Input: part model. Units: mm. Frame: model coordinates. A direction names the side the tool comes from. Coordinates: 2 decimals unless noted, no trailing zeros. Write each loop counter-clockwise with the first axis right and the second up, starting at its lowest first coordinate (ties: lowest second). Pieces come first, ordered by that corner, then holes. Notation, with made-up numbers: (-36.5, -12) - (5.5, -12) arc R23 cw to (5.5, 0) - close; hole circle Ø1 at (25, 50). An arc over 180 degrees is marked (long way). Use a Markdown table: item, result. Add a question column.
Q1. Pin query (flat end, axial travel): P1, Ø7.5, axis at x = 6, y = -5, coming from the -Z side. Return the tip coordinate at first contact, or that it passes through.
Q2. Material intervals for probe 1 along X at (y, z) = (-23.5, 1.35); probe 2 along Y at (x, z) = (6, 1.2); probe 3 along Y at (x, z) = (26, 2.1), sorted ascending. Write a range as from..to.
Q3. Set-up query: faces 5 (the face through (1, -42, 1)), 6 (the face through (23, -12, 1)), 7 (the face through (12.341, -22.308, 2.065)). Return all of +Z, -Z, +X, -X, +Y, -Y with unobstructed straight access to the full face (end or side cutting, diameter ignored); none if empty.
Q4. Section query A-A (z = 0.4). Return the cut outline in (x, y), then the cut area to 3 significant figures.
Q5. Section query B-B (y = -19). Return the cut outline in (x, z).
Q6. Section query C-C (x = 6). Return the cut outline in (y, z).
Q7. Mould query, pull axis Y, two halves, no side actions, for faces 1 (the face through (16, -44, 1)), 2 (the face through (17.8, -21.7, 2.6)), 3 (the face through (1, -2, 1)), 4 (the face through (18.6, -12.57, 1.32)). Classes: released by +Y, released by -Y, zero draft, split by the parting line, or undercut.
Q8. Section query D-D (x = 18.5). Return the cut outline in (y, z), then the cut area to 3 significant figures.
from build123d import *

# Parameters (mm, degrees)
F0_W     = 32
F0_H     = 44
F1_DEPTH = 2.6
F2_R     = 2.35
F3_DEPTH = 2.6
F5_DEPTH = 44.001
F6_R     = 5
F8_DEPTH = 2.601


with BuildPart() as f1:
    # F0 (on Top) → F1 (new body)
    with BuildSketch(Plane.XY):
        with Locations((16, -22)):
            Rectangle(F0_W, F0_H)
    extrude(amount=F1_DEPTH)

    # F2 (on face) → F3 (cut, through all)
    with BuildSketch(Plane.XY.offset(2.6)):
        with Locations((6, -5)):
            Circle(F2_R)
        with Locations((6, -39)):
            Circle(F2_R)
        with Locations((26, -39)):
            Circle(F2_R)
        with Locations((26, -5)):
            Circle(F2_R)
    extrude(amount=-F3_DEPTH, mode=Mode.SUBTRACT)

    # F4 (on face) → F5 (cut, through all)
    with BuildSketch(Plane.XZ.offset(44)):
        with BuildLine():
            Line((12.494805, 2.6), (11.505195, 2.6))
            Line((11.505195, 2.6), (11.807748, 1.544873))
            ThreePointArc((11.807748, 1.544873), (12, 1.4), (12.192252, 1.544873))
            Line((12.192252, 1.544873), (12.494805, 2.6))
        make_face()
    extrude(amount=-F5_DEPTH, mode=Mode.SUBTRACT)

    # F6
    f6_edges = [f1.edges().sort_by_distance(p)[0] for p in [
        (0, -44, 1.3),
        (32, -44, 1.3),
        (32, 0, 1.3),
        (0, 0, 1.3),
    ]]
    fillet(f6_edges, radius=F6_R)

    # F7 (on face) → F8 (cut, through all)
    with BuildSketch(Plane.XY.offset(2.6)):
        with BuildLine():
            Line((8, -30), (8, -14))
            ThreePointArc((8, -14), (6, -12), (4, -14))
            Line((4, -14), (4, -30))
            ThreePointArc((4, -30), (6, -32), (8, -30))
        make_face()
        with BuildLine():
            Line((25, -12), (20, -12))
            ThreePointArc((20, -12), (18.585786, -12.585786), (18, -14))
            Line((18, -14), (18, -30))
            ThreePointArc((18, -30), (18.585786, -31.414214), (20, -32))
            Line((20, -32), (25, -32))
            ThreePointArc((25, -32), (26.414214, -31.414214), (27, -30))
            Line((27, -30), (27, -14))
            ThreePointArc((27, -14), (26.414214, -12.585786), (25, -12))
        make_face()
    extrude(amount=-F8_DEPTH, mode=Mode.SUBTRACT)


solid = f1.part
Values follow:
| question | item | result |
|---|---|---|
| 1 | P1 | z = 0 |
| 2 | probe 1 | 0..4, 8..18, 27..32 |
| 2 | probe 2 | -44..-41.35, -36.65..-32, -12..-7.35, -2.65..0 |
| 2 | probe 3 | -44..-41.35, -36.65..-31.73, -12.27..-7.35, -2.65..0 |
| 3 | face 5 | +Z, -Z, -X, -Y |
| 3 | face 6 | +Z, -Z |
| 3 | face 7 | +Z, +Y, -Y |
| 4 | outline | (0, -39) arc R5 ccw to (5, -44) - (27, -44) arc R5 ccw to (32, -39) - (32, -5) arc R5 ccw to (27, 0) - (5, 0) arc R5 ccw to (0, -5) - close; hole circle Ø4.7 at (6, -39); hole circle Ø4.7 at (6, -5); hole (4, -30) arc R2 ccw to (8, -30) - (8, -14) arc R2 ccw to (4, -14) - close; hole (18, -30) arc R2 ccw to (20, -32) - (25, -32) arc R2 ccw to (27, -30) - (27, -14) arc R2 ccw to (25, -12) - (20, -12) arc R2 ccw to (18, -14) - close; hole circle Ø4.7 at (26, -39); hole circle Ø4.7 at (26, -5) |
| 4 | area | 1,060 mm2 |
| 5 | outline | (0, 0) - (4, 0) - (4, 2.6) - (0, 2.6) - close; (8, 0) - (18, 0) - (18, 2.6) - (12.49, 2.6) - (12.19, 1.54) arc R0.2 cw to (11.81, 1.54) - (11.51, 2.6) - (8, 2.6) - close; (27, 0) - (32, 0) - (32, 2.6) - (27, 2.6) - close |
| 6 | outline | (-44, 0) - (-41.35, 0) - (-41.35, 2.6) - (-44, 2.6) - close; (-36.65, 0) - (-32, 0) - (-32, 2.6) - (-36.65, 2.6) - close; (-12, 0) - (-7.35, 0) - (-7.35, 2.6) - (-12, 2.6) - close; (-2.65, 0) - (0, 0) - (0, 2.6) - (-2.65, 2.6) - close |
| 7 | face 1 | released by -Y |
| 7 | face 2 | zero draft |
| 7 | face 3 | released by +Y |
| 7 | face 4 | undercut |
| 8 | outline | (-44, 0) - (-31.32, 0) - (-31.32, 2.6) - (-44, 2.6) - close; (-12.68, 0) - (0, 0) - (0, 2.6) - (-12.68, 2.6) - close |
| 8 | area | 65.9 mm2 |
